Could you check a few things on this model? Use its own coordinates, in mm. A direction names the side the tool comes from. Give positions to 0.01 mm unless a question says otherwise; leave off trailing zeros. Loops run counter-clockwise (first coordinate to the right, second up) from the corner with the lowest first, then second, coordinate; pieces in that order, holes last.
1. Thinking about a two-plate mould opening in X: for faces 5 (the flat face through (-59.402, -17.123, -67.984)), 6 (the flat face through (-66.13, -9.235, -82.347)), 7 (the flat face through (76.404, -17.167, -67.499)), which applies, +X half, -X half, draft (parallel to the pull), parting line (faces both ways), or undercut?
2. Imagine slicing it at A-A (y = -10.5). List the corners of the cut face in (x, z) for me, plus the area to 3 significant figures.
3. For P1, Ø5, axis at x = -40.5, z = -47, coming from the -Y side (3 decimals); P2, Ø1.5, axis at y = -2.5, z = -61, coming from the +X side, each with a flat end and sliding along its axis, tell me the tip position at first contact or that it passes through.
4. For faces 1 (the flat face through (64.54, -9.28, -79.6)), 2 (the flat face through (47.205, -17.167, -80.425)), 3 (the flat face through (58.993, -17.123, -68.165)), 4 (the flat face through (17, 0, -29)), which set-ups out of +Z, -Z, +X, -X, +Y, -Y let a thin tool reach every point of the face, with its end or its side?
5. I need wall thicknesses on line 1 along Y through (x, z) = (43, -46) (3 decimals); line 2 along X through (y, z) = (-2.5, -19.5); line 3 along X through (y, z) = (-9.5, -75.5). Which ranges of each line are inside material? Lowest first, please.
6. Imagine slicing it at B-B (z = -55.5). List the corners of the cut face in (x, y) for me (3 decimals).
7. Imagine slicing it at C-C (z = 50.5). List the corners of the cut face in (x, y) for me (3 decimals), plus the area to 3 significant figures.
8. Imagine slicing it at D-D (x = 9). List the corners of the cut face in (y, z) for me (3 decimals).
```python
from build123d import *

# Parameters (mm, degrees)
F1_DEPTH = 3.175
F3_DEPTH = 15.5575
F4_W     = 31.932119
F4_H     = 3.175
F5_DEPTH = 12.7
F6_W     = 31.932119
F6_H     = 3.175
F7_DEPTH = 12.7


with BuildPart() as f1:
    # F0 (on Front) → F1 (new body)
    with BuildSketch(Plane.XZ):
        Polygon((0, 63.5), (0, 0), (51.326439, -88.9), (80.525518, -75.974289), align=None)
        Polygon((-51.326439, -88.9), (0, 0), (0, 63.5), (-80.525518, -75.974289), align=None)
    extrude(amount=F1_DEPTH)

    # F2 (on face) → F3 (join)
    with BuildSketch(Plane.XZ.offset(3.175)):
        Polygon((-78.938018, -73.224658), (-80.525518, -75.974289), (-51.326439, -88.9), (-49.738939, -86.150369), align=None)
        Polygon((49.738939, -86.150369), (51.326439, -88.9), (80.525518, -75.974289), (78.938018, -73.224658), align=None)
    extrude(amount=F3_DEPTH)

    # F4 (on face) → F5 (join)
    with BuildSketch(Plane(origin=(-40.037708, 0, -90.444865), x_dir=(0.914411, 0, -0.404787), z_dir=(0.404787, 0, 0.914411))):
        with Locations((-26.575328, -17.145)):
            Rectangle(F4_W, F4_H)
    extrude(amount=F5_DEPTH)

    # F6 (on face) → F7 (join)
    with BuildSketch(Plane(origin=(40.037708, 0, -90.444865), x_dir=(0.914411, 0, 0.404787), z_dir=(-0.404787, 0, 0.914411))):
        with Locations((26.575328, -17.145)):
            Rectangle(F6_W, F6_H)
    extrude(amount=F7_DEPTH)


solid = f1.part
```
Derived:
1. face 5: undercut
1. face 6: -X half
1. face 7: +X half
2. outline: (-80.53, -75.97) - (-51.33, -88.9) - (-49.74, -86.15) - (-78.94, -73.22) - close; (49.74, -86.15) - (51.33, -88.9) - (80.53, -75.97) - (78.94, -73.22) - close
2. area: 202 mm2
3. P1: stops at y = -3.175
3. P2: stops at x = 72.31
4. face 1: +Z
4. face 2: -Z, -Y
4. face 3: +Z, -Y
4. face 4: +Z, -Z, +X, -X, +Y
5. line 1: y = -3.175 to 0
5. line 2: x = -47.92 to -11.26, 11.26 to 47.92
5. line 3: x = -80.25 to -73.8, 73.8 to 80.25
6. outline: (-68.705, -3.175) - (-32.043, -3.175) - (-32.043, 0) - (-68.705, 0) - close; (32.043, -3.175) - (68.705, -3.175) - (68.705, 0) - (32.043, 0) - close
7. outline: (-7.506, -3.175) - (7.506, -3.175) - (7.506, 0) - (-7.506, 0) - close
7. area: 47.7 mm2
8. outline: (-3.175, -15.588) - (0, -15.588) - (0, 47.912) - (-3.175, 47.912) - close
